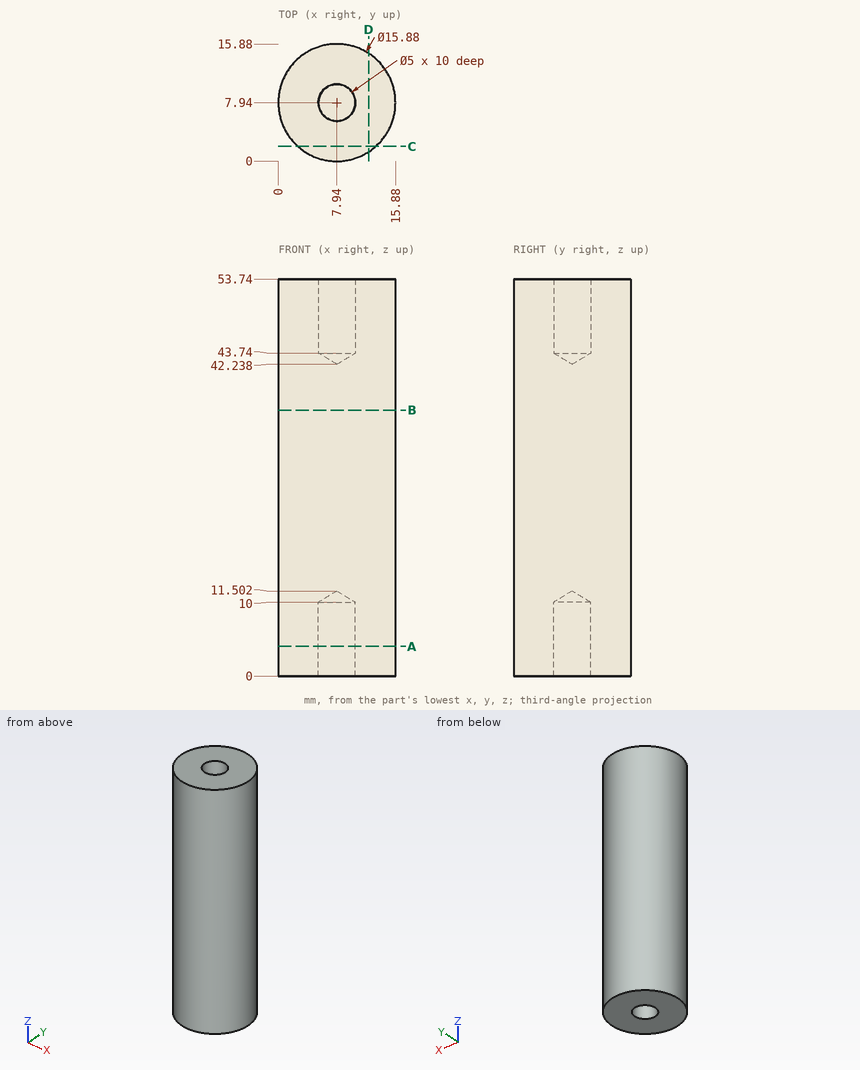
The drawing under review shows one solid part. Ordinate dimensions are in mm from its lowest x, y, z. Round coordinates to 2 decimals unless told otherwise and drop trailing zeros. Write each loop counter-clockwise with the first axis right and the second up, starting at its lowest first coordinate (ties: lowest second). Pieces come first, ordered by that corner, then holes.
(1) We need section C-C on y = 2. Give the boundary of the cut face in (x, z), and give its area (3 significant figures).
(2) Insertion check: pin 1 (2 mm diameter, centred on x = 10, z = 8, fed in from +Y); pin 2 (3 mm diameter, centred on x = 3.5, z = 15, fed in from -Y); pin 3 (5 mm diameter, centred on y = 13.5, z = 43.5, fed in from -X). Each pin has a flat end and moves straight along its axis. Give the tip position at first contact, or say it passes through.
(3) We need section A-A on z = 4. Give the boundary of the cut face in (x, y).
(4) Wall thickness on L1, parallel to Y at x = 7.94, z = 51; L2, parallel to Y at x = 8.75, z = 46 (1 decimal); L3, parallel to Y at x = 8.25, z = 19.5: over which ranges is each line inside the solid? List them lowest first.
(5) We need section D-D on x = 12.25. Give the boundary of the cut face in (y, z).
(6) We need section B-B on z = 36. Give the boundary of the cut face in (x, y).
Findings below:
1. outline: (2.67, 0) - (13.21, 0) - (13.21, 53.74) - (2.67, 53.74) - close
1. area: 566 mm2
2. pin 1: stops at y = 15.81
2. pin 2: stops at y = 0.56
2. pin 3: stops at x = 0.61
3. outline: circle Ø15.88 at (7.94, 7.94); hole circle Ø5 at (7.94, 7.94)
4. L1: y = 0 to 5.44, 10.44 to 15.88
4. L2: y = 0 to 5.6, 10.3 to 15.8
4. L3: y = 0.01 to 15.87
5. outline: (1.27, 0) - (14.61, 0) - (14.61, 53.74) - (1.27, 53.74) - close
6. outline: circle Ø15.88 at (7.94, 7.94)
